Here's the drawing with two shaded views (mm, measured from the low corner). I have some questions. A direction names the side the tool comes from. Give positions to 0.01 mm unless a question says otherwise; leave off trailing zeros. Order: outer loops, then holes, each group sorted by start corner. A loop starts at its lowest first (then second) coordinate and runs counter-clockwise, first axis right, second up. Notation, with made-up numbers: M 17,82.25 L 26,82.25 A14 cw 26,101.25 Z; hole C -39,69.5 d9. An arc over 180 degrees is marked long. Use a Markdown table: item, result. Add a question column.
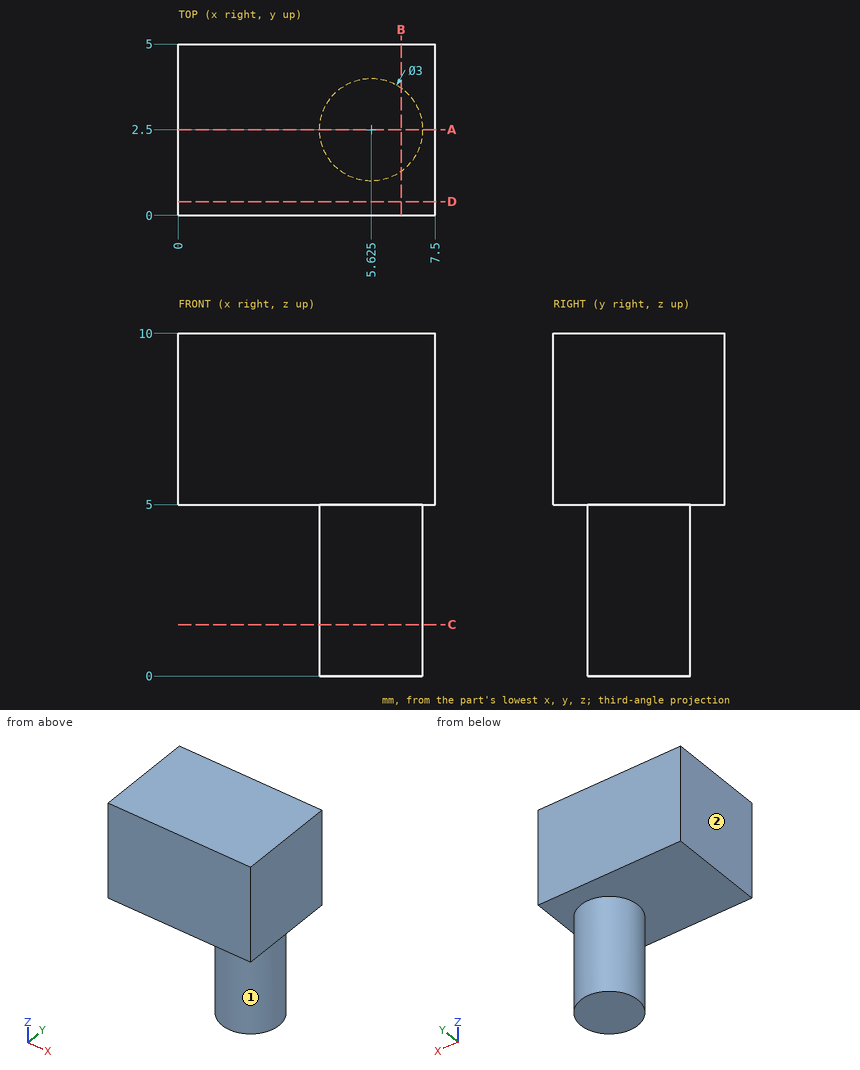
1. If we section it at B-B, the plane x = 6.5: List the corners of the cut face in (y, z) for me.
2. If we section it at C-C, the plane z = 1.5: List the corners of the cut face in (x, y) for me (3 decimals).
3. On a 3-axis mill with a long thin cutter (end or side, diameter ignored), from which of +Z, -Z, +X, -X, +Y, -Y can I reach the whole of each face in a straight line? I mean the marked faces 1 and 2. Say none if no direction works.
4. I need wall thicknesses on L1, parallel to Z at x = 2.75, y = 2; L2, parallel to X at y = 2.4, z = 4.5; L3, parallel to X at y = 2.1, z = 1.75. Which ranges of each line are inside material? Lowest first, please. Write a range as [from, to].
5. If we section it at D-D, the plane y = 0.4: List the corners of the cut face in (x, z) for me.
6. If we section it at A-A, the plane y = 2.5: List the corners of the cut face in (x, z) for me (3 decimals), then the cut area to 3 significant figures.
7. Will this pin go through, and if not, where does the flat tip stop? pin 1 (2 mm diameter, centred on y = 4, z = 2, fed in from -X).
Geometry results:
| question | item | result |
|---|---|---|
| 1 | outline | M 0,5 L 1.28,5 L 1.28,0 L 3.72,0 L 3.72,5 L 5,5 L 5,10 L 0,10 Z |
| 2 | outline | C 5.625,2.5 d3 |
| 3 | face 1 | -Z |
| 3 | face 2 | +Z, -Z, -X, +Y, -Y |
| 4 | L1 | z = [5, 10] |
| 4 | L2 | x = [4.13, 7.12] |
| 4 | L3 | x = [4.18, 7.07] |
| 5 | outline | M 0,5 L 7.5,5 L 7.5,10 L 0,10 Z |
| 6 | outline | M 0,5 L 4.125,5 L 4.125,0 L 7.125,0 L 7.125,5 L 7.5,5 L 7.5,10 L 0,10 Z |
| 6 | area | 52.5 mm^2 |
| 7 | pin 1 | stops at x = 4.21 |
